Source: CAD feature listing. Evaluate the final solid. Frame: model axes, mm. Round coordinates to 2 decimals unless told otherwise and drop trailing zeros. Write each loop counter-clockwise with the first axis right and the second up, starting at its lowest first coordinate (ties: lowest second). Pieces come first, ordered by that corner, then holes. Notation, with made-up numbers: M 30,79 L 59,79 A19 cw 59,97 Z; hole C 63.25,22 d10. An arc over 180 degrees is marked long. Answer in a Markdown table with one row per item. Add a question column.
Item 1: Cut plane A-A on z = 0. Return loops of the section in (x, y).
Item 2: Material intervals for probe 1 along Y at (x, z) = (-0.8, -15); probe 2 along Z at (x, y) = (-0.85, 16); probe 3 along Z at (x, y) = (-0.15, 12), sorted ascending.
Item 3: Mould query, pull axis Z, two halves, no side actions, for faces 1 (the face through (-0.592, -5.362, -12.932)), 2 (the face through (-1, 0, 19)), 3 (the face through (0, 13, 9)), 4 (the face through (-1, 0, -19)). Classes: released by +Z, released by -Z, zero draft, split by the parting line, or undercut.
Item 4: Cut plane C-C on z = -12.5. Return loops of the section in (x, y).
Item 5: Cut plane D-D on x = -0.25. Return loops of the section in (y, z) (3 decimals), and give its area (3 significant figures).
from build123d import *

# Parameters (mm, degrees)
CROQUIS2_W        = 38
CROQUIS2_H        = 38
CROQUIS2_R        = 14
CROQUIS2_R_2      = 3
BRIDA_BASE1_DEPTH = 1.2


# Sheet-metal steps are written as plain solids
with BuildPart() as part:
    # Croquis2 → Brida base1 (new body)
    with BuildSketch(Plane(origin=(0, 0, 0), x_dir=(0, 0, -1), z_dir=(1, 0, 0))):
        Rectangle(CROQUIS2_W, CROQUIS2_H)
        Circle(CROQUIS2_R, mode=Mode.SUBTRACT)
        with Locations((-14.085, -14.085)):
            Circle(CROQUIS2_R_2, mode=Mode.SUBTRACT)
        with Locations((-14.085, 14.085)):
            Circle(CROQUIS2_R_2, mode=Mode.SUBTRACT)
        with Locations((14.085, 14.085)):
            Circle(CROQUIS2_R_2, mode=Mode.SUBTRACT)
        with Locations((14.085, -14.085)):
            Circle(CROQUIS2_R_2, mode=Mode.SUBTRACT)
    extrude(amount=-BRIDA_BASE1_DEPTH)


solid = part.part
Results below:
| question | item | result |
|---|---|---|
| 1 | outline | M -1.2,-19 L 0,-19 L 0,-14 L -1.2,-14 Z; M -1.2,14 L 0,14 L 0,19 L -1.2,19 Z |
| 2 | probe 1 | -19 to -16.94, -11.23 to 11.23, 16.94 to 19 |
| 2 | probe 2 | -19 to -16.39, -11.78 to 11.78, 16.39 to 19 |
| 2 | probe 3 | -19 to -16.24, -11.93 to -7.21, 7.21 to 11.93, 16.24 to 19 |
| 3 | face 1 | undercut |
| 3 | face 2 | released by +Z |
| 3 | face 3 | zero draft |
| 3 | face 4 | released by -Z |
| 4 | outline | M -1.2,-19 L 0,-19 L 0,-16.63 L -1.2,-16.63 Z; M -1.2,-11.54 L 0,-11.54 L 0,-6.3 L -1.2,-6.3 Z; M -1.2,6.3 L 0,6.3 L 0,11.54 L -1.2,11.54 Z; M -1.2,16.63 L 0,16.63 L 0,19 L -1.2,19 Z |
| 5 | outline | M -19,-19 L 19,-19 L 19,19 L -19,19 Z; hole C -14.085,-14.085 d6; hole C -14.085,14.085 d6; hole C 0,0 d28; hole C 14.085,-14.085 d6; hole C 14.085,14.085 d6 |
| 5 | area | 715 mm2 |
